from build123d import *

# Parameters (mm, degrees)
SKETCH1_W           = 152.4
SKETCH1_H           = 50.8
SKETCH1_R           = 3.175
BOSS_EXTRUDE1_DEPTH = 6.35


with BuildPart() as part:
    # Sketch1 → Boss-Extrude1 (new body)
    with BuildSketch(Plane(origin=(0, 0, 0), x_dir=(1, 0, 0), z_dir=(0, 1, 0))):
        Rectangle(SKETCH1_W, SKETCH1_H)
        with Locations(Location((31.75, 19.05, 0), (0, 0, 270))):
            Circle(SKETCH1_R, mode=Mode.SUBTRACT)
        with Locations(Location((44.45, 19.05, 0), (0, 0, 270))):
            Circle(SKETCH1_R, mode=Mode.SUBTRACT)
        with Locations(Location((57.15, 19.05, 0), (0, 0, 270))):
            Circle(SKETCH1_R, mode=Mode.SUBTRACT)
        with Locations(Location((31.75, 6.35, 0), (0, 0, 270))):
            Circle(SKETCH1_R, mode=Mode.SUBTRACT)
        with Locations(Location((44.45, 6.35, 0), (0, 0, 270))):
            Circle(SKETCH1_R, mode=Mode.SUBTRACT)
        with Locations(Location((57.15, 6.35, 0), (0, 0, 270))):
            Circle(SKETCH1_R, mode=Mode.SUBTRACT)
        with Locations(Location((69.85, 6.35, 0), (0, 0, 270))):
            Circle(SKETCH1_R, mode=Mode.SUBTRACT)
        with Locations(Location((31.75, -6.35, 0), (0, 0, 270))):
            Circle(SKETCH1_R, mode=Mode.SUBTRACT)
        with Locations(Location((44.45, -6.35, 0), (0, 0, 270))):
            Circle(SKETCH1_R, mode=Mode.SUBTRACT)
        with Locations(Location((57.15, -6.35, 0), (0, 0, 270))):
            Circle(SKETCH1_R, mode=Mode.SUBTRACT)
        with Locations(Location((69.85, -6.35, 0), (0, 0, 270))):
            Circle(SKETCH1_R, mode=Mode.SUBTRACT)
        with Locations(Location((31.75, -19.05, 0), (0, 0, 270))):
            Circle(SKETCH1_R, mode=Mode.SUBTRACT)
        with Locations(Location((69.85, 19.05, 0), (0, 0, 270))):
            Circle(SKETCH1_R, mode=Mode.SUBTRACT)
        with Locations(Location((44.45, -19.05, 0), (0, 0, 270))):
            Circle(SKETCH1_R, mode=Mode.SUBTRACT)
        with Locations(Location((57.15, -19.05, 0), (0, 0, 270))):
            Circle(SKETCH1_R, mode=Mode.SUBTRACT)
        with Locations(Location((69.85, -19.05, 0), (0, 0, 270))):
            Circle(SKETCH1_R, mode=Mode.SUBTRACT)
        with BuildLine():
            Line((-69.85, 22.225), (19.05, 22.225))
            ThreePointArc((19.05, 22.225), (22.225, 19.05), (19.05, 15.875))
            Line((19.05, 15.875), (-69.85, 15.875))
            ThreePointArc((-69.85, 15.875), (-73.025, 19.05), (-69.85, 22.225))
        make_face(mode=Mode.SUBTRACT)
        with BuildLine():
            Line((19.05, 3.175), (-69.85, 3.175))
            ThreePointArc((-69.85, 3.175), (-73.025, 6.35), (-69.85, 9.525))
            Line((-69.85, 9.525), (19.05, 9.525))
            ThreePointArc((19.05, 9.525), (22.225, 6.35), (19.05, 3.175))
        make_face(mode=Mode.SUBTRACT)
        with BuildLine():
            Line((19.05, -9.525), (-69.85, -9.525))
            ThreePointArc((-69.85, -9.525), (-73.025, -6.35), (-69.85, -3.175))
            Line((-69.85, -3.175), (19.05, -3.175))
            ThreePointArc((19.05, -3.175), (22.225, -6.35), (19.05, -9.525))
        make_face(mode=Mode.SUBTRACT)
        with BuildLine():
            Line((19.05, -22.225), (-69.85, -22.225))
            ThreePointArc((-69.85, -22.225), (-73.025, -19.05), (-69.85, -15.875))
            Line((-69.85, -15.875), (19.05, -15.875))
            ThreePointArc((19.05, -15.875), (22.225, -19.05), (19.05, -22.225))
        make_face(mode=Mode.SUBTRACT)
    extrude(amount=BOSS_EXTRUDE1_DEPTH)


solid = part.part
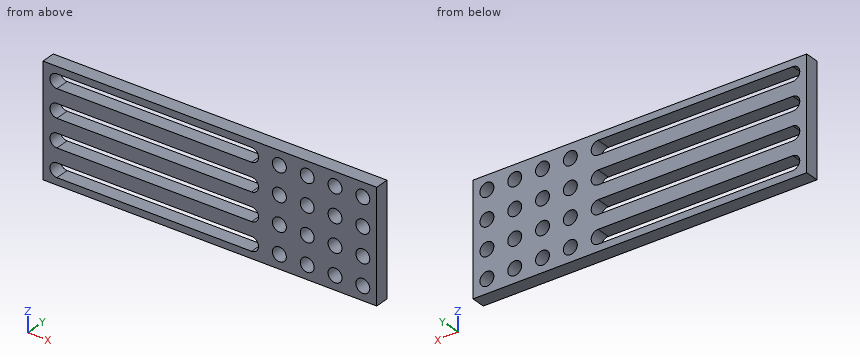
Input: part model. Units: mm. Frame: model coordinates. Give positions to 0.01 mm unless a question says otherwise; leave off trailing zeros. Write each loop counter-clockwise with the first axis right and the second up, starting at its lowest first coordinate (ties: lowest second). Pieces come first, ordered by that corner, then holes.
Q1. Material intervals for probe 1 along X at (y, z) = (2, -6.35) (3 decimals); probe 2 along Z at (x, y) = (-42.5, 4.5) (3 decimals); probe 3 along Z at (x, y) = (58, 4.75), sorted ascending.
Q2. Section B-B, the plane z = -6.35. Output: boundary loops of the cut face in (x, y) (3 decimals).
Q3. Section D-D, the plane x = 20.5. Output: boundary loops of the cut face in (y, z), plus the area to 3 significant figures.
Q4. Section C-C, the plane y = 4. State how many separate pieces and enclosed holes the cut face has, plus the area to 3 significant figures.
Q5. Section A-A, the plane x = 57.15. Output: boundary loops of the cut face in (y, z) (3 decimals), plus the area to 3 significant figures.
Filled in:
1. probe 1: x = -76.2 to -73.025, 22.225 to 28.575, 34.925 to 41.275, 47.625 to 53.975, 60.325 to 66.675, 73.025 to 76.2
1. probe 2: z = -25.4 to -22.225, -15.875 to -9.525, -3.175 to 3.175, 9.525 to 15.875, 22.225 to 25.4
1. probe 3: z = -25.4 to -22.11, -15.99 to -9.41, -3.29 to 3.29, 9.41 to 15.99, 22.11 to 25.4
2. outline: (-76.2, 0) - (-73.025, 0) - (-73.025, 6.35) - (-76.2, 6.35) - close; (22.225, 0) - (28.575, 0) - (28.575, 6.35) - (22.225, 6.35) - close; (34.925, 0) - (41.275, 0) - (41.275, 6.35) - (34.925, 6.35) - close; (47.625, 0) - (53.975, 0) - (53.975, 6.35) - (47.625, 6.35) - close; (60.325, 0) - (66.675, 0) - (66.675, 6.35) - (60.325, 6.35) - close; (73.025, 0) - (76.2, 0) - (76.2, 6.35) - (73.025, 6.35) - close
3. outline: (0, -25.4) - (6.35, -25.4) - (6.35, -21.87) - (0, -21.87) - close; (0, -16.23) - (6.35, -16.23) - (6.35, -9.17) - (0, -9.17) - close; (0, -3.53) - (6.35, -3.53) - (6.35, 3.53) - (0, 3.53) - close; (0, 9.17) - (6.35, 9.17) - (6.35, 16.23) - (0, 16.23) - close; (0, 21.87) - (6.35, 21.87) - (6.35, 25.4) - (0, 25.4) - close
3. area: 179 mm2
4. separate pieces: 1
4. enclosed holes: 20
4. area: 4,850 mm2
5. outline: (0, -25.4) - (6.35, -25.4) - (6.35, -22.225) - (0, -22.225) - close; (0, -15.875) - (6.35, -15.875) - (6.35, -9.525) - (0, -9.525) - close; (0, -3.175) - (6.35, -3.175) - (6.35, 3.175) - (0, 3.175) - close; (0, 9.525) - (6.35, 9.525) - (6.35, 15.875) - (0, 15.875) - close; (0, 22.225) - (6.35, 22.225) - (6.35, 25.4) - (0, 25.4) - close
5. area: 161 mm2
